The model under review builds one solid part; all positions refer to its coordinate system, in mm. A direction names the side the tool comes from. Round coordinates to 2 decimals unless told otherwise and drop trailing zeros. Write each loop counter-clockwise with the first axis right and the second up, starting at its lowest first coordinate (ties: lowest second). Pieces come first, ordered by that corner, then holes. Notation, with made-up numbers: (27, 67.5) - (53, 67.5) arc R6 cw to (53, 73.5) - close; hole circle Ø1 at (-14.75, 20). An arc over 180 degrees is marked (long way). Return JSON: item names as keys, results as strings.
Autodesk Fusion 360 part; units mm, degrees
sketch "Sketch1" plane through (0, 0, 0) normal (0, 1, 0) x (1, 0, 0)
  line L0 (0, 0) -> (0, 830)
  line L1 (0, 830) -> (200, 830)
  line L2 (0, 0) -> (770, 0)
  line L3 (770, 0) -> (200, 830)
  dimension "d1" = 830
  dimension "d2" = 770
extrude "Extrude1" add sketch "Sketch1" along normal blind 11
sketch "Sketch2" plane through (0, 11, 0) normal (0, 1, 0) x (-1, 0, 0)
  line L0 (0, 0) -> (-770, 0)
  line L1 (-770, 0) -> (-200, -830)
  line L2 (-200, -830) -> (0, -830)
  line L3 (0, -830) -> (0, 0)
  arc A0 (-167.9783, -725.6164) -> (-256.5823, -748.2599) centre (-183.687, -848.8237) ccw
  arc A1 (-171.646, -754.3836) -> (-167.9783, -725.6164) centre (-169.8121, -740) ccw
  arc A2 (-171.646, -754.3836) -> (-239.5623, -771.7401) centre (-183.687, -848.8237) ccw
  arc A3 (-256.5823, -748.2599) -> (-239.5623, -771.7401) centre (-248.0723, -760) ccw
  arc A4 (-169.8121, -740) -> (-248.0723, -760) centre (-183.687, -848.8237) ccw construction
  arc A5 (-277.8741, -599.4877) -> (-346.9644, -617.3771) centre (-282.9401, -722.2833) ccw
  arc A6 (-277.8741, -599.4877) -> (-276.6787, -570.5123) centre (-277.2764, -585) ccw
  arc A7 (-276.6787, -570.5123) -> (-362.0718, -592.6229) centre (-282.9401, -722.2833) ccw
  arc A8 (-362.0718, -592.6229) -> (-346.9644, -617.3771) centre (-354.5181, -605) ccw
  arc A9 (-277.2764, -585) -> (-354.5181, -605) centre (-282.9401, -722.2833) ccw construction
  arc A10 (-370.6712, -454.4432) -> (-446.4891, -472.3442) centre (-381.6102, -577.6218) ccw
  arc A11 (-370.6712, -454.4432) -> (-368.1059, -425.5568) centre (-369.3886, -440) ccw
  arc A12 (-368.1059, -425.5568) -> (-461.7037, -447.6558) centre (-381.6102, -577.6218) ccw
  arc A13 (-461.7037, -447.6558) -> (-446.4891, -472.3442) centre (-454.0964, -460) ccw
  arc A14 (-369.3886, -440) -> (-454.0964, -460) centre (-381.6102, -577.6218) ccw construction
  arc A15 (-470.9702, -309.4832) -> (-546.4851, -327.592) centre (-477.6426, -448.1642) ccw
  arc A16 (-470.9702, -309.4832) -> (-469.5765, -280.5168) centre (-470.2734, -295) ccw
  arc A17 (-469.5765, -280.5168) -> (-560.8643, -302.408) centre (-477.6426, -448.1642) ccw
  arc A18 (-560.8643, -302.408) -> (-546.4851, -327.592) centre (-553.6747, -315) ccw
  arc A19 (-470.2734, -295) -> (-553.6747, -315) centre (-477.6426, -448.1642) ccw construction
  arc A20 (-574.3852, -164.4572) -> (-645.4659, -182.2316) centre (-583.2764, -279.9159) ccw
  arc A21 (-574.3852, -164.4572) -> (-572.1585, -135.5428) centre (-573.2718, -150) ccw
  arc A22 (-572.1585, -135.5428) -> (-661.0401, -157.7684) centre (-583.2764, -279.9159) ccw
  arc A23 (-661.0401, -157.7684) -> (-645.4659, -182.2316) centre (-653.253, -170) ccw
  arc A24 (-573.2718, -150) -> (-653.253, -170) centre (-583.2764, -279.9159) ccw construction
  line L4 (-573.2718, -164.5) -> (-373.7749, -164.5)
  arc A25 (-373.7749, -164.5) -> (-373.7749, -135.5) centre (-373.7749, -150) ccw
  line L5 (-373.7749, -135.5) -> (-573.2718, -135.5)
  arc A26 (-573.2718, -135.5) -> (-573.2718, -164.5) centre (-573.2718, -150) ccw
  line L6 (-573.2718, -150) -> (-373.7749, -150) construction
  line L7 (-470.2734, -309.5) -> (-277.2764, -309.5)
  arc A27 (-277.2764, -309.5) -> (-277.2764, -280.5) centre (-277.2764, -295) ccw
  line L8 (-277.2764, -280.5) -> (-470.2734, -280.5)
  arc A28 (-470.2734, -280.5) -> (-470.2734, -309.5) centre (-470.2734, -295) ccw
  line L9 (-470.2734, -295) -> (-277.2764, -295) construction
  line L10 (-369.3886, -454.5) -> (-200, -454.5)
  arc A29 (-200, -454.5) -> (-200, -425.5) centre (-200, -440) ccw
  line L11 (-200, -425.5) -> (-369.3886, -425.5)
  arc A30 (-369.3886, -425.5) -> (-369.3886, -454.5) centre (-369.3886, -440) ccw
  line L12 (-369.3886, -440) -> (-200, -440) construction
  line L13 (-277.2764, -599.5) -> (-200, -599.5)
  arc A31 (-200, -599.5) -> (-200, -570.5) centre (-200, -585) ccw
  line L14 (-200, -570.5) -> (-277.2764, -570.5)
  arc A32 (-277.2764, -570.5) -> (-277.2764, -599.5) centre (-277.2764, -585) ccw
  line L15 (-277.2764, -585) -> (-200, -585) construction
  dimension "d13" = 90
  dimension "d14" = 245
  dimension "d15" = 390
  dimension "d16" = 390
  dimension "d17" = 535
  dimension "d18" = 535
  dimension "d19" = 680
  dimension "d20" = 680
  dimension "d21" = 29
  dimension "d22" = 29
  dimension "d23" = 29
  dimension "d24" = 29
  dimension "d25" = 29
  dimension "d26" = 20
  dimension "d27" = 20
  dimension "d28" = 20
  dimension "d29" = 20
  dimension "d30" = 20
  dimension "d31" = 29
  dimension "d32" = 29
  dimension "d33" = 29
  dimension "d40" = 29
extrude "Extrude2" cut sketch "Sketch2" against normal blind 12 contours L1 A20 A22 A23 L5 A26 | L1 A20 A23 | L1 A0 A3 | L1 A0 A1 A2 A3 | L1 A15 A17 A18 L8 A28 | L1 A15 A18 | A21 A22 L5 A26 | A21 A22 L4 A25 L5 | L1 A5 A8 | L1 A5 A7 A8 L14 A32 | L1 A10 A12 A13 L11 A30 | L1 A10 A13 | A16 A17 L8 A28 | A16 A17 L7 A27 L8 | A6 A7 L14 A32 | A11 A12 L11 A30 | A11 A12 L10 A29 L11
fillet "Fillet1" radius 50 1 edges at (0, 5.5, -830)
fillet "Fillet2" radius 50 1 edges at (200, 5.5, -830)
fillet "Fillet3" radius 50 1 edges at (0, 5.5, 0)
fillet "Fillet4" radius 20 1 edges at (770, 5.5, 0)
extrude "Extrude3" cut sketch "Sketch2" against normal blind 12 contours A6 A7 L13 A31 L14
sketch "Sketch3" plane through (0, 11, 0) normal (0, 1, 0) x (-1, 0, 0)
  line L0 (-276.9849, -570.5) -> (-200, -570.5)
  arc A0 (-200, -599.5) -> (-200, -570.5) centre (-200, -585) ccw
  line L1 (-200, -599.5) -> (-277.2764, -599.5)
  arc A1 (-277.8741, -599.4877) -> (-277.2764, -599.5) centre (-277.2764, -585) ccw
  arc A2 (-277.8741, -599.4877) -> (-346.2962, -616.9722) centre (-282.9401, -722.2833) ccw
  line L2 (-346.2962, -616.9722) -> (-256.2832, -748.0438)
  arc A3 (-167.9783, -725.6164) -> (-256.2832, -748.0438) centre (-183.687, -848.8237) ccw
  arc A4 (-171.646, -754.3836) -> (-167.9783, -725.6164) centre (-169.8121, -740) ccw
  arc A5 (-171.646, -754.3836) -> (-239.5623, -771.7401) centre (-183.687, -848.8237) ccw
  arc A6 (-239.8637, -771.9528) -> (-239.5623, -771.7401) centre (-248.0723, -760) ccw
  line L3 (-239.8637, -771.9528) -> (-214.8987, -808.3054)
  arc A7 (-214.8987, -808.3054) -> (-173.6821, -830) centre (-173.6821, -780) ccw
  line L4 (-173.6821, -830) -> (-50, -830)
  arc A8 (-50, -830) -> (0, -780) centre (-50, -780) ccw
  line L5 (0, -780) -> (0, -50)
  arc A9 (0, -50) -> (-50, 0) centre (-50, -50) ccw
  line L6 (-50, 0) -> (-732.003, 0)
  arc A10 (-732.003, 0) -> (-748.4896, -31.3221) centre (-732.003, -20) ccw
  line L7 (-748.4896, -31.3221) -> (-661.4616, -158.0472)
  arc A11 (-661.0401, -157.7684) -> (-661.4616, -158.0472) centre (-653.253, -170) ccw
  arc A12 (-572.7291, -135.5) -> (-661.0401, -157.7684) centre (-583.2764, -279.9159) ccw
  line L8 (-572.7291, -135.5) -> (-373.7749, -135.5)
  arc A13 (-373.7749, -164.5) -> (-373.7749, -135.5) centre (-373.7749, -150) ccw
  line L9 (-373.7749, -164.5) -> (-573.2718, -164.5)
  arc A14 (-574.3852, -164.4572) -> (-573.2718, -164.5) centre (-573.2718, -150) ccw
  arc A15 (-574.3852, -164.4572) -> (-645.0388, -181.961) centre (-583.2764, -279.9159) ccw
  line L10 (-645.0388, -181.961) -> (-561.8833, -303.0472)
  arc A16 (-560.8643, -302.408) -> (-561.8833, -303.0472) centre (-553.6747, -315) ccw
  arc A17 (-469.9326, -280.5) -> (-560.8643, -302.408) centre (-477.6426, -448.1642) ccw
  line L11 (-469.9326, -280.5) -> (-277.2764, -280.5)
  arc A18 (-277.2764, -309.5) -> (-277.2764, -280.5) centre (-277.2764, -295) ccw
  line L12 (-277.2764, -309.5) -> (-470.2734, -309.5)
  arc A19 (-470.9702, -309.4832) -> (-470.2734, -309.5) centre (-470.2734, -295) ccw
  arc A20 (-470.9702, -309.4832) -> (-545.4348, -326.9984) centre (-477.6426, -448.1642) ccw
  line L13 (-545.4348, -326.9984) -> (-462.3049, -448.0472)
  arc A21 (-461.7037, -447.6558) -> (-462.3049, -448.0472) centre (-454.0964, -460) ccw
  arc A22 (-368.762, -425.5) -> (-461.7037, -447.6558) centre (-381.6102, -577.6218) ccw
  line L14 (-368.762, -425.5) -> (-200, -425.5)
  arc A23 (-200, -454.5) -> (-200, -425.5) centre (-200, -440) ccw
  line L15 (-200, -454.5) -> (-369.3886, -454.5)
  arc A24 (-370.6712, -454.4432) -> (-369.3886, -454.5) centre (-369.3886, -440) ccw
  arc A25 (-370.6712, -454.4432) -> (-445.8766, -471.9692) centre (-381.6102, -577.6218) ccw
  line L16 (-445.8766, -471.9692) -> (-362.7266, -593.0472)
  arc A26 (-362.0718, -592.6229) -> (-362.7266, -593.0472) centre (-354.5181, -605) ccw
  arc A27 (-276.9849, -570.5) -> (-362.0718, -592.6229) centre (-282.9401, -722.2833) ccw
  circle A28 centre (-40, -790) radius 13.9
  circle A29 centre (-60, -60) radius 13.9
  circle A30 centre (-682.712, -40) radius 13.9
  circle A31 centre (-50, -415) radius 13.9
  dimension "d43" = 27.8
  dimension "d44" = 40
  dimension "d45" = 40
  dimension "d46" = 27.8
  dimension "d47" = 27.8
  dimension "d48" = 60
  dimension "d49" = 60
  dimension "d50" = 40
  dimension "d51" = 27.8
  dimension "d52" = 50
  dimension "d53" = 415
extrude "Extrude4" cut sketch "Sketch3" against normal blind 12 contours A28 | A29 | A30 | A31
(1) Wall thickness on line 1 (Z direction, x = 50, y = 7.5); line 2 (Z direction, x = 494, y = 5.75); line 3 (Z direction, x = 425, y = 2.5): over which ranges is each line inside the solid? List them lowest first.
Filled in:
{"line 1": "z = -830 to -799.65, -780.35 to -428.9, -401.1 to -69.65, -50.35 to 0", "line 2": "z = -401.89 to -310.29, -281.12 to -164.5, -135.5 to 0", "line 3": "z = -502.37 to -461.82, -431.25 to -309.5, -280.5 to -164.5, -135.5 to 0"}
(2) Add section C-C (z = -632.5). Write out the cut boundary in (x, y), plus the area to 3 significant figures.
Filled in:
{"outline": "(0, 0) - (335.63, 0) - (335.63, 11) - (0, 11) - close", "area": "3,690 mm2"}
(3) Clearance check with flat-ended pins moving along their axes: pin 1 Ø2 at (x, y) = (536.5, 6.5) entering from +Z; pin 2 Ø25 at (x, z) = (50, -415) entering from -Y; pin 3 Ø3.5 at (x, y) = (264.5, 6.5) entering from -Z; pin 4 Ø3.5 at (x, y) = (345.5, 5) entering from -Z. State where each tip first meets the part, or that it passes through.
Filled in:
{"pin 1": "stops at z = 0", "pin 2": "passes through", "pin 3": "stops at z = -738.63", "pin 4": "stops at z = -620.68"}
(4) Add section A-A (x = 519.5). Write out the cut boundary in (y, z).
Filled in:
{"outline": "(0, -364.76) - (11, -364.76) - (11, -315.78) - (0, -315.78) - close; (0, -285.63) - (11, -285.63) - (11, -164.5) - (0, -164.5) - close; (0, -135.5) - (11, -135.5) - (11, 0) - (0, 0) - close"}
(5) Add section B-B (y = 7.5). Give the number of separate pieces and of enclosed holes in the cut face, plus the area to 3 significant figures.
Filled in:
{"separate pieces": "1", "enclosed holes": "4", "area": "366,000 mm2"}
(6) For faces 5 (the flat face through (227.56, 5.42, -789.87)), 6 (the cylindrical face through (516.31, 5.577, -284.838)), list the 3-axis set-ups (+Z, -Z, +X, -X, +Y, -Y) from which the entire face can be reached by the end or side of a thin tool; tool diameter is ignored.
Filled in:
{"face 5": "-Z, +X, +Y, -Y", "face 6": "+Y, -Y"}
(7) Mouldability with a two-part tool opening along X and no side actions: class faces 1 (the flat face through (287, 11, -329)), 2 (the cylindrical face through (14.258, 5.577, -15.036)), 3 (the cylindrical face through (213.628, 5.577, -728.282)), 4 (the cylindrical face through (197.27, 5.577, -824.086)) as released by +X, released by -X, zero draft, split by the parting line, or undercut.
Filled in:
{"face 1": "zero draft", "face 2": "released by -X", "face 3": "undercut", "face 4": "released by +X"}
